```python
from build123d import *
from OCP.BRepFilletAPI import BRepFilletAPI_MakeChamfer

# Parameters (mm, degrees)
ESQUISSE1_W             = 35
ESQUISSE1_H             = 15
BOSS_EXTRU_1_DEPTH      = 3
ESQUISSE4_R             = 3
ENL_V_MAT_EXTRU_1_DEPTH = 39.19685851
CHANFREIN1_SIZE         = 4
ENL_V_MAT_EXTRU_2_DEPTH = 39.19685851
ESQUISSE6_W             = 5
ESQUISSE6_H             = 15
BOSS_EXTRU_2_DEPTH      = 7
ESQUISSE7_W             = 23
ESQUISSE7_H             = 2.2
ENL_V_MAT_EXTRU_3_DEPTH = 40.37003937
CHANFREIN2_SIZE         = 6
CHANFREIN2_SIZE2        = 2.183821406
ESQUISSE8_R             = 1.5
ENL_V_MAT_EXTRU_4_DEPTH = 7


with BuildPart() as part:
    # Esquisse1 → Boss.-Extru.1 (new body)
    with BuildSketch(Plane.XY):
        with Locations((17.5, 7.5)):
            Rectangle(ESQUISSE1_W, ESQUISSE1_H)
    extrude(amount=BOSS_EXTRU_1_DEPTH)

    # Esquisse4 → Enlèv. mat.-Extru.1 (cut, through all)
    with BuildSketch(Plane.XY.offset(3)):
        with Locations((6, 7.5)):
            Circle(ESQUISSE4_R)
    extrude(amount=-ENL_V_MAT_EXTRU_1_DEPTH, mode=Mode.SUBTRACT)

    # Chanfrein1
    chanfrein1_edges = [part.edges().sort_by_distance(p)[0] for p in [
        (0, 15, 1.5),
        (0, 0, 1.5),
    ]]
    chamfer(chanfrein1_edges, length=CHANFREIN1_SIZE)

    # Esquisse5 → Enlèv. mat.-Extru.2 (cut, through all)
    with BuildSketch(Plane(origin=(0, 0, 0), x_dir=(-1, 0, 0), z_dir=(0, 0, -1))):
        with BuildLine():
            Line((-19, 5.9), (-25, 5.9))
            ThreePointArc((-25, 5.9), (-26.6, 7.5), (-25, 9.1))
            Line((-25, 9.1), (-19, 9.1))
            ThreePointArc((-19, 9.1), (-17.4, 7.5), (-19, 5.9))
        make_face()
    extrude(amount=-ENL_V_MAT_EXTRU_2_DEPTH, mode=Mode.SUBTRACT)

    # Esquisse6 → Boss.-Extru.2 (add)
    with BuildSketch(Plane(origin=(0, 0, 0), x_dir=(-1, 0, 0), z_dir=(0, 0, -1))):
        with Locations((-32.5, 7.5)):
            Rectangle(ESQUISSE6_W, ESQUISSE6_H)
    extrude(amount=BOSS_EXTRU_2_DEPTH)

    # Esquisse7 → Enlèv. mat.-Extru.3 (cut, through all)
    with BuildSketch(Plane(origin=(0, 0, -7), x_dir=(-1, 0, 0), z_dir=(0, 0, -1))):
        with Locations((-23.5, 1.1)):
            Rectangle(ESQUISSE7_W, ESQUISSE7_H)
        with Locations((-23.5, 13.9)):
            Rectangle(ESQUISSE7_W, ESQUISSE7_H)
    extrude(amount=-ENL_V_MAT_EXTRU_3_DEPTH, mode=Mode.SUBTRACT)

    # Chanfrein2: one chamfer whose edges measure the first distance from different faces: ONE call of the kernel's chamfer builder (chamfer() names one face for all edges)
    chanfrein2_edges_1 = [part.edges().sort_by_distance(p)[0] for p in [
        (12, 0, 1.5),
    ]]
    chanfrein2_side_1 = [part.faces().sort_by_distance(p)[0] for p in [
        (8, 0, 1.5),
    ]]
    chanfrein2_edges_2 = [part.edges().sort_by_distance(p)[0] for p in [
        (12, 15, 1.5),
    ]]
    chanfrein2_side_2 = [part.faces().sort_by_distance(p)[0] for p in [
        (8, 15, 1.5),
    ]]
    chanfrein2 = BRepFilletAPI_MakeChamfer(part.part.solid().wrapped)
    for e in chanfrein2_edges_1:
        chanfrein2.Add(CHANFREIN2_SIZE, CHANFREIN2_SIZE2, e.wrapped, chanfrein2_side_1[0].wrapped)  # the first distance lies on this face
    for e in chanfrein2_edges_2:
        chanfrein2.Add(CHANFREIN2_SIZE, CHANFREIN2_SIZE2, e.wrapped, chanfrein2_side_2[0].wrapped)  # the first distance lies on this face
    add(Compound.cast(chanfrein2.Shape()), mode=Mode.REPLACE)

    # Esquisse8 → Enlèv. mat.-Extru.4 (cut)
    with BuildSketch(Plane.ZY.offset(-30)):
        with Locations((-4, 7.5)):
            Circle(ESQUISSE8_R)
    extrude(amount=-ENL_V_MAT_EXTRU_4_DEPTH, mode=Mode.SUBTRACT)


solid = part.part
```
Check sheet for the modelled part. Datum: model origin and axes. Units: mm. A direction names the side the tool comes from. Round coordinates to 2 decimals unless told otherwise and drop trailing zeros. Order: outer loops, then holes, each group sorted by start corner. A loop starts at its lowest first (then second) coordinate and runs counter-clockwise, first axis right, second up. Notation, with made-up numbers: (65.25, 68.25) -> (105.25, 68.25) arc R21 ccw to (105.25, 89.25) -> close; hole circle Ø11 at (65, 28). An arc over 180 degrees is marked (long way). One line per item, written item: value. Start each with the question number.
Q1. Set-up check for faces 4 (the face through (26.2, 2.2, 0.2)), 5 (the face through (17.4, 7.5, 1.5)), 6 (the face through (15, 8, 0)): record each of +Z, -Z, +X, -X, +Y, -Y from which the full face is reachable in a straight line by a thin tool's end or side.
Q2. Gauge pin test, flat ends, axial feed: pin 1 Ø1.5 at (x, z) = (21, 1.5) entering from +Y; pin 2 Ø4 at (y, z) = (8, -4.5) entering from -X; pin 3 Ø7.5 at (x, y) = (18, 10) entering from -Z; pin 4 Ø5 at (x, y) = (6, 7.5) entering from +Z. Record the tip position at first contact, or that the pin passes through.
Q3. Cross-section at A-A (y = 7.5). Record the boundary of the cut face in (x, z), and give its area (3 significant figures).
Q4. Mould release check, pull along X, two halves, no side actions. Record for faces 1 (the face through (17, 8, 3)), 2 (the face through (0, 7, 1)), 3 (the face through (26.6, 7.5, 1.5)): pulls with the +X half, pulls with the -X half, needs draft (parallel to the pull), parting line crosses it, or undercut.
Q5. Cross-section at B-B (z = -4). Record the boundary of the cut face in (x, y), and give its area (3 significant figures).
Q6. Cross-section at D-D (z = 0.5). Give the number of separate pieces and of enclosed holes in the cut face, and give its area (3 significant figures).
Q7. Cross-section at C-C (x = 19.5). Record the boundary of the cut face in (y, z), and give its area (3 significant figures).
Q8. Thickness scan on line 1 (Y direction, x = 32.8, z = -4); line 2 (Y direction, x = 6, z = 0.6); line 3 (Z direction, x = 14.5, y = 11.25). Record the ranges inside material, lowest first.
Completed:
1. face 4: +Z, -Z, +X, -Y
1. face 5: +Z, -Z
1. face 6: -Z, -X, +Y, -Y
2. pin 1: stops at y = 12.8
2. pin 2: stops at x = 30
2. pin 3: stops at z = 0
2. pin 4: passes through
3. outline: (0, 0) -> (3, 0) -> (3, 3) -> (0, 3) -> close; (9, 0) -> (17.4, 0) -> (17.4, 3) -> (9, 3) -> close; (26.6, 0) -> (30, 0) -> (30, -2.5) -> (35, -2.5) -> (35, 3) -> (26.6, 3) -> close; (30, -7) -> (35, -7) -> (35, -5.5) -> (30, -5.5) -> close
3. area: 79.4 mm²
4. face 1: needs draft
4. face 2: pulls with the -X half
4. face 3: undercut
5. outline: (30, 2.2) -> (35, 2.2) -> (35, 6) -> (30, 6) -> close; (30, 9) -> (35, 9) -> (35, 12.8) -> (30, 12.8) -> close
5. area: 38.0 mm²
6. separate pieces: 1
6. enclosed holes: 2
6. area: 339 mm²
7. outline: (2.2, 0) -> (5.9, 0) -> (5.9, 3) -> (2.2, 3) -> close; (9.1, 0) -> (12.8, 0) -> (12.8, 3) -> (9.1, 3) -> close
7. area: 22.2 mm²
8. line 1: y = 2.2 to 6, 9 to 12.8
8. line 2: y = 0 to 4.5, 10.5 to 15
8. line 3: z = 0 to 3
